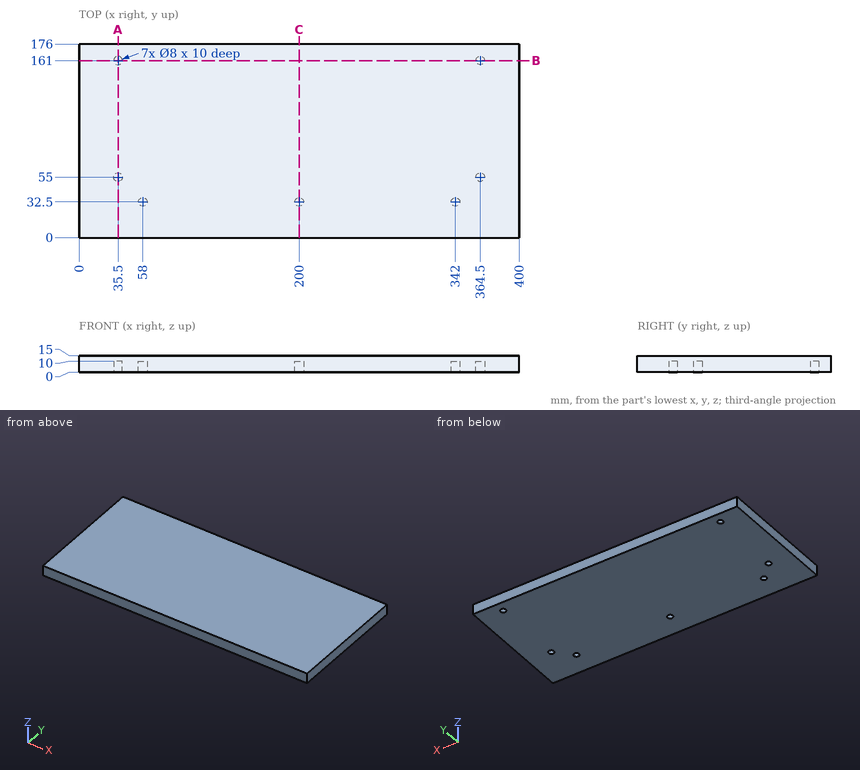
Could you check a few things on this drawing? It's one solid part, dimensions in mm from its lowest x, y, z. Coordinates: 2 decimals unless noted, no trailing zeros. Loops run counter-clockwise (first coordinate to the right, second up) from the corner with the lowest first, then second, coordinate; pieces in that order, holes last.
1. Imagine slicing it at B-B (y = 161). Please give me the cut outline in (x, z).
2. For P1, Ø5, axis at x = 364.5, y = 55, coming from the -Z side, with a flat end and sliding along its axis, tell me the tip position at first contact or that it passes through.
3. I need wall thicknesses on L1, parallel to X at y = 161, z = 7.75; L2, parallel to Y at x = 35.5, z = 4.75; L3, parallel to Y at x = 342, z = 7. Which ranges of each line are inside material? Lowest first, please.
4. Imagine slicing it at C-C (x = 200). Please give me the cut outline in (y, z), and give its area (3 significant figures).
5. Imagine slicing it at A-A (x = 35.5). Please give me the cut outline in (y, z), and give its area (3 significant figures).
Computed values:
1. outline: (0, 0) - (31.5, 0) - (31.5, 10) - (39.5, 10) - (39.5, 0) - (360.5, 0) - (360.5, 10) - (368.5, 10) - (368.5, 0) - (400, 0) - (400, 15) - (0, 15) - close
2. P1: stops at z = 10
3. L1: x = 0 to 31.5, 39.5 to 360.5, 368.5 to 400
3. L2: y = 0 to 51, 59 to 157, 165 to 176
3. L3: y = 0 to 28.5, 36.5 to 176
4. outline: (0, 0) - (28.5, 0) - (28.5, 10) - (36.5, 10) - (36.5, 0) - (176, 0) - (176, 15) - (0, 15) - close
4. area: 2,560 mm2
5. outline: (0, 0) - (51, 0) - (51, 10) - (59, 10) - (59, 0) - (157, 0) - (157, 10) - (165, 10) - (165, 0) - (176, 0) - (176, 15) - (0, 15) - close
5. area: 2,480 mm2
